Source: CAD feature listing. Evaluate the final solid. Frame: model axes, mm. A direction names the side the tool comes from. Give positions to 0.01 mm unless a question says otherwise; leave off trailing zeros. Loops run counter-clockwise (first coordinate to the right, second up) from the corner with the lowest first, then second, coordinate; pieces in that order, holes last. Notation, with made-up numbers: M 49.5,20.25 L 67.5,20.25 A31 cw 67.5,50.25 Z; hole C 77.5,-11.75 d2. An arc over 180 degrees is marked long. Put each result on its own line as item: value.
from build123d import *

# Parameters (mm, degrees)
F0_W     = 127
F0_H     = 43.0744847506
F1_DEPTH = 127


with BuildPart() as f1:
    # F0 (on Front) → F1 (new body)
    with BuildSketch(Plane.XZ):
        with Locations((0, 41.9627576247)):
            Rectangle(F0_W, F0_H)
        with Locations((0, -41.9627576247)):
            Rectangle(F0_W, F0_H)
        with BuildLine():
            Line((63.5, -20.4255152494), (63.5, 0))
            Line((63.5, 0), (60.0370731576, 0))
            ThreePointArc((60.0370731576, 0), (50.5451090429, -11.7795835352), (37.0166287351, -5.0093404391))
            ThreePointArc((37.0166287351, -5.0093404391), (19.5052616542, -17.06006857), (3.7896064307, -2.7462219024))
            ThreePointArc((3.7896064307, -2.7462219024), (-14.0682122313, -16.6503534924), (-29.3976705132, 0))
            Line((-29.3976705132, 0), (-29.8486748192, 0))
            ThreePointArc((-29.8486748192, 0), (-46.2897717953, -16.4410969761), (-62.7308687714, 0))
            Line((-62.7308687714, 0), (-63.5, 0))
            Line((-63.5, 0), (-63.5, -20.4255152494))
            Line((-63.5, -20.4255152494), (63.5, -20.4255152494))
        make_face()
        with BuildLine():
            Line((63.5, 0), (63.5, 20.4255152494))
            Line((63.5, 20.4255152494), (-63.5, 20.4255152494))
            Line((-63.5, 20.4255152494), (-63.5, 0))
            Line((-63.5, 0), (-62.7308687714, 0))
            ThreePointArc((-62.7308687714, 0), (-46.2897717953, 16.4410969761), (-29.8486748192, 0))
            Line((-29.8486748192, 0), (-29.3976705132, 0))
            ThreePointArc((-29.3976705132, 0), (-14.0682122313, 16.6503534924), (3.7896064307, 2.7462219024))
            ThreePointArc((3.7896064307, 2.7462219024), (19.5052616542, 17.06006857), (37.0166287351, 5.0093404391))
            ThreePointArc((37.0166287351, 5.0093404391), (50.5451090429, 11.7795835352), (60.0370731576, 0))
            Line((60.0370731576, 0), (63.5, 0))
        make_face()
        with BuildLine():
            ThreePointArc((-29.3976705132, 0), (-14.0682122313, -16.6503534924), (3.7896064307, -2.7462219024))
            ThreePointArc((3.7896064307, -2.7462219024), (3.6232234507, -1.3775887394), (3.5676420141, 0))
            Line((3.5676420141, 0), (0, 0))
            ThreePointArc((0, 0), (-12.6904081553, -12.6904081553), (-25.3808163106, 0))
            Line((-25.3808163106, 0), (-29.3976705132, 0))
        make_face()
        with BuildLine():
            ThreePointArc((3.5676420141, 0), (3.6232234507, 1.3775887394), (3.7896064307, 2.7462219024))
            ThreePointArc((3.7896064307, 2.7462219024), (-14.0682122313, 16.6503534924), (-29.3976705132, 0))
            Line((-29.3976705132, 0), (-25.3808163106, 0))
            Line((-25.3808163106, 0), (0, 0))
            Line((0, 0), (3.5676420141, 0))
        make_face()
        with BuildLine():
            ThreePointArc((-29.8486748192, 0), (-46.2897717953, 16.4410969761), (-62.7308687714, 0))
            Line((-62.7308687714, 0), (-58.8593184948, 0))
            Line((-58.8593184948, 0), (-33.7202250957, 0))
            Line((-33.7202250957, 0), (-29.8486748192, 0))
        make_face()
        with BuildLine():
            ThreePointArc((35.9265762941, 0), (36.2022411907, 2.563284317), (37.0166287351, 5.0093404391))
            ThreePointArc((37.0166287351, 5.0093404391), (19.5052616542, 17.06006857), (3.7896064307, 2.7462219024))
            ThreePointArc((3.7896064307, 2.7462219024), (3.9599453371, 1.377804076), (4.0168542025, 0))
            Line((4.0168542025, 0), (7.8559666872, 0))
            Line((7.8559666872, 0), (33.4785059094, 0))
            Line((33.4785059094, 0), (35.9265762941, 0))
        make_face()
        with BuildLine():
            Line((57.8924268484, 0), (60.0370731576, 0))
            ThreePointArc((60.0370731576, 0), (50.5451090429, 11.7795835352), (37.0166287351, 5.0093404391))
            ThreePointArc((37.0166287351, 5.0093404391), (37.5782401442, 2.5326021424), (37.7668305826, 0))
            Line((37.7668305826, 0), (38.0712226033, 0))
            Line((38.0712226033, 0), (57.8924268484, 0))
        make_face()
        with BuildLine():
            ThreePointArc((37.0166287351, -5.0093404391), (50.5451090429, -11.7795835352), (60.0370731576, 0))
            Line((60.0370731576, 0), (57.8924268484, 0))
            ThreePointArc((57.8924268484, 0), (47.9818247259, -9.9106021225), (38.0712226033, 0))
            Line((38.0712226033, 0), (37.7668305826, 0))
            ThreePointArc((37.7668305826, 0), (37.5782401442, -2.5326021424), (37.0166287351, -5.0093404391))
        make_face()
        with BuildLine():
            ThreePointArc((35.9265762941, 0), (36.2022411907, -2.563284317), (37.0166287351, -5.0093404391))
            ThreePointArc((37.0166287351, -5.0093404391), (37.5782401442, -2.5326021424), (37.7668305826, 0))
            Line((37.7668305826, 0), (35.9265762941, 0))
        make_face()
        with BuildLine():
            ThreePointArc((37.7668305826, 0), (37.5782401442, 2.5326021424), (37.0166287351, 5.0093404391))
            ThreePointArc((37.0166287351, 5.0093404391), (36.2022411907, 2.563284317), (35.9265762941, 0))
            Line((35.9265762941, 0), (37.7668305826, 0))
        make_face()
        with BuildLine():
            ThreePointArc((3.7896064307, -2.7462219024), (19.5052616542, -17.06006857), (37.0166287351, -5.0093404391))
            ThreePointArc((37.0166287351, -5.0093404391), (36.2022411907, -2.563284317), (35.9265762941, 0))
            Line((35.9265762941, 0), (33.4785059094, 0))
            ThreePointArc((33.4785059094, 0), (20.6672362983, -12.8112696111), (7.8559666872, 0))
            Line((7.8559666872, 0), (4.0168542025, 0))
            ThreePointArc((4.0168542025, 0), (3.9599453371, -1.377804076), (3.7896064307, -2.7462219024))
        make_face()
        with BuildLine():
            Line((-58.8593184948, 0), (-62.7308687714, 0))
            ThreePointArc((-62.7308687714, 0), (-46.2897717953, -16.4410969761), (-29.8486748192, 0))
            Line((-29.8486748192, 0), (-33.7202250957, 0))
            ThreePointArc((-33.7202250957, 0), (-46.2897717953, -12.5695466995), (-58.8593184948, 0))
        make_face()
    extrude(amount=F1_DEPTH)


solid = f1.part
1. Section query B-B (y = -33). Output: boundary loops of the cut face in (x, z), plus the area to 3 significant figures.
Found:
outline: M -63.5,-63.5 L 63.5,-63.5 L 63.5,63.5 L -63.5,63.5 Z; hole M -58.86,0 A12.57 ccw -33.72,0 Z; hole M -25.38,0 A12.69 ccw 0,0 Z; hole M 3.79,-2.75 A16.71 ccw 3.79,2.75 A17.1 ccw Z; hole M 7.86,0 A12.81 ccw 33.48,0 Z; hole M 38.07,0 A9.91 ccw 57.89,0 Z
area: 15,200 mm^2
2. Draft query along Z for faces 1 (the flat face through (63.5, -63, -1)), 2 (the flat face through (-1, -63, -63.5)), 3 (the flat face through (-13, -63, 0)). Return one class per face: pulls with the +Z half, pulls with the -Z half, needs draft (parallel to the pull), parting line crosses it, or undercut.
Found:
face 1: needs draft
face 2: pulls with the -Z half
face 3: undercut
3. Section query C-C (x = 48.5). Output: boundary loops of the cut face in (y, z).
Found:
outline: M -127,-63.5 L 0,-63.5 L 0,-9.9 L -127,-9.9 Z; M -127,0 L 0,0 L 0,63.5 L -127,63.5 Z
4. Section query A-A (x = 21). Output: boundary loops of the cut face in (y, z).
Found:
outline: M -127,-63.5 L 0,-63.5 L 0,-12.81 L -127,-12.81 Z; M -127,0 L 0,0 L 0,63.5 L -127,63.5 Z
5. Material intervals for line 1 (Z direction, x = -14.5, y = -101); line 2 (Z direction, x = 30, y = -25), sorted ascending. Write a range as from..to.
Found:
line 1: -63.5..-12.56, 0..63.5
line 2: -63.5..-8.78, 0..63.5
6. Access query for faces 4 (the flat face through (48, -63, 0)), 5 (the flat face through (-1, 0, 1)). Directions: +Z, -Z, +X, -X, +Y, -Y. A direction counts if a zero-diameter tool reaches every point of the face in a straight line with its end or side. Return the directions, or none.
Found:
face 4: +Y, -Y
face 5: +Z, -Z, +X, -X, +Y
